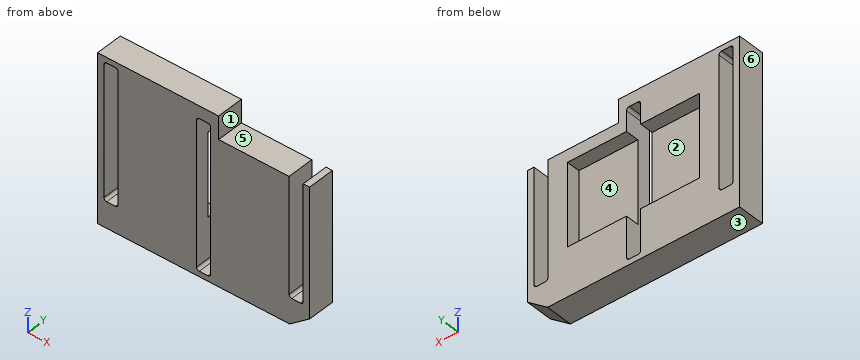
```python
from build123d import *

# Parameters (mm, degrees)
BOSS_EXTRUDE1_DEPTH = 10
FILLET1_R           = 1
SKETCH2_W           = 21.86553483
SKETCH2_H           = 30.5
CUT_EXTRUDE1_DEPTH  = 5
MIRROR1_DEPTH       = 10
MIRROR1_2_OUTLINE_W = 21.86553483
MIRROR1_2_OUTLINE_H = 30.5
MIRROR1_2_DEPTH     = 5
SKETCH6_W           = 43.680332617
SKETCH6_H           = 16.249834628
CUT_EXTRUDE2_DEPTH  = 10


# Read off the part's stored shape, not the designer's step: Mirror1
with BuildPart() as part:
    # Sketch1 → Boss-Extrude1 (new body)
    with BuildSketch(Plane(origin=(0, 0, 0), x_dir=(1, 0, 0), z_dir=(0, 1, 0))):
        Polygon((-5, 57.097150921), (34.3, 57.097150921), (34.3, 55.097150921), (31.675, 55.097150921), (31.675, 52.597150921), (31.675, 2.599340873), (31.675, 0.099340873), (34.3, 0.099340873), (34.3, -4.5), (-5, -4.5), align=None)
        Polygon((-2.625, 45), (-2.625, 0), (-2.625, -2.5), (0, -2.5), (2.625, -2.5), (2.625, 0), (2.625, 45), (2.625, 47.5), (0, 47.5), (-2.625, 47.5), align=None, mode=Mode.SUBTRACT)
    extrude(amount=BOSS_EXTRUDE1_DEPTH)

    # Fillet1
    fillet1_edges = [part.edges().sort_by_distance(p)[0] for p in [
        (31.675, 5, -55.097150921),
        (31.675, 5, -0.099340873),
        (-2.625, 5, -47.5),
        (-2.625, 5, 2.5),
        (2.625, 5, 2.5),
        (2.625, 5, -47.5),
    ]]
    fillet(fillet1_edges, radius=FILLET1_R)

    # Sketch2 → Cut-Extrude1 (cut)
    with BuildSketch(Plane(origin=(0, 10, 0), x_dir=(1, 0, 0), z_dir=(0, 1, 0))):
        with Locations((20.742232585, 23.8519351)):
            Rectangle(SKETCH2_W, SKETCH2_H)
    extrude(amount=-CUT_EXTRUDE1_DEPTH, mode=Mode.SUBTRACT)

    # Mirror1 outline → Mirror1 (add)
    with BuildSketch(Plane(origin=(0, 0, 0), x_dir=(1, 0, 0), z_dir=(0, 1, 0))):
        with BuildLine():
            ThreePointArc((35.925, 55.097150921), (36.632106781, 54.804257702), (36.925, 54.097150921))
            Line((36.925, 54.097150921), (36.925, 39.1019351))
            Line((36.925, 39.1019351), (58.79053483, 39.1019351))
            Line((58.79053483, 39.1019351), (58.79053483, 8.6019351))
            Line((58.79053483, 8.6019351), (36.925, 8.6019351))
            Line((36.925, 8.6019351), (36.925, 1.099340873))
            ThreePointArc((36.925, 1.099340873), (36.632106781, 0.392234092), (35.925, 0.099340873))
            Line((35.925, 0.099340873), (34.3, 0.099340873))
            Line((34.3, 0.099340873), (34.3, -4.5))
            Line((34.3, -4.5), (73.6, -4.5))
            Line((73.6, -4.5), (73.6, 57.097150921))
            Line((73.6, 57.097150921), (34.3, 57.097150921))
            Line((34.3, 57.097150921), (34.3, 55.097150921))
            Line((34.3, 55.097150921), (35.925, 55.097150921))
        make_face()
        with BuildLine():
            Line((70.225, -2.5), (66.975, -2.5))
            ThreePointArc((66.975, -2.5), (66.267893219, -2.207106781), (65.975, -1.5))
            Line((65.975, -1.5), (65.975, 46.5))
            ThreePointArc((65.975, 46.5), (66.267893219, 47.207106781), (66.975, 47.5))
            Line((66.975, 47.5), (70.225, 47.5))
            ThreePointArc((70.225, 47.5), (70.932106781, 47.207106781), (71.225, 46.5))
            Line((71.225, 46.5), (71.225, -1.5))
            ThreePointArc((71.225, -1.5), (70.932106781, -2.207106781), (70.225, -2.5))
        make_face(mode=Mode.SUBTRACT)
    extrude(amount=MIRROR1_DEPTH)

    # Mirror1 2 outline → Mirror1 2 (add)
    with BuildSketch(Plane(origin=(0, 0, 0), x_dir=(1, 0, 0), z_dir=(0, 1, 0))):
        with Locations((47.857767415, 23.8519351)):
            Rectangle(MIRROR1_2_OUTLINE_W, MIRROR1_2_OUTLINE_H)
    extrude(amount=MIRROR1_2_DEPTH)

    # Sketch6 → Cut-Extrude2 (cut)
    with BuildSketch(Plane(origin=(0, 10, 0), x_dir=(1, 0, 0), z_dir=(0, 1, 0))):
        with Locations((61.699631479, -4.127511542)):
            Rectangle(SKETCH6_W, SKETCH6_H)
        Polygon((66.193799085, 57.097150921), (73.6, 51.534362723), (73.6, 57.097150921), align=None)
    extrude(amount=-CUT_EXTRUDE2_DEPTH, mode=Mode.SUBTRACT)


solid = part.part
```
For this review, take the finished solid that the model builds, in its own axes (mm). Face numbers are marked on the shaded views. A direction names the side the tool comes from. Coordinates: 2 decimals unless noted, no trailing zeros. Loops run counter-clockwise (first coordinate to the right, second up) from the corner with the lowest first, then second, coordinate; pieces in that order, holes last. Notation, with made-up numbers: (-15.75, -34) - (19.25, -34) arc R34 cw to (19.25, 0) - close; hole circle Ø8 at (69.25, 70.25). An arc over 180 degrees is marked (long way). Use one line per item in the form item = value. Start each with the question number.
1) Take a section at C-C (y = 1). State how many separate pieces and enclosed holes the cut face has, plus the area to 3 significant figures.
2) For pin 1 (24 mm diameter, centred on x = 22.5, z = -25, fed in from +Y), flat-tipped, find the tip position at first contact; note if it passes through.
3) For the marked faces 4, 5 and 6, list the 3-axis set-ups (+Z, -Z, +X, -X, +Y, -Y) from which the entire face can be reached by the end or side of a thin tool; tool diameter is ignored.
4) Take a section at A-A (z = -7.5). State the section outline as (x, y) points (3 decimals), plus the area to 4 significant figures.
5) To check wall thickness, follow probe 1 along X at (y, z) = (3, -8) (3 decimals); probe 2 along X at (y, z) = (9.5, -20) (3 decimals); probe 3 along X at (y, z) = (7, -3.5) (3 decimals). State the ranges of each line that lie inside material, in increasing order. Write a range as from..to.
6) Draft analysis for pull direction Z (two halves, no side actions). For the marked faces 1, 2 and 3, state which applies: released by +Z, released by -Z, zero draft, split by the parting line, or undercut.
7) Take a section at D-D (z = -18). State the section outline as (x, y) points (3 decimals).
8) Take a section at B-B (x = 50). State the section outline as (y, z) points.
From the geometry:
q1.separate_pieces = 1
q1.enclosed_holes = 2
q1.area = 3,760 mm2
q2.pin_1 = 5
q3.face_4 = +Y
q3.face_5 = +Z, +X, +Y, -Y
q3.face_6 = +Z, -Z, -X, +Y, -Y
q4.outline = (-5, 0) - (-2.625, 0) - (-2.625, 10) - (-5, 10) - close; (2.625, 0) - (31.675, 0) - (31.675, 10) - (2.625, 10) - close; (36.925, 0) - (65.975, 0) - (65.975, 10) - (36.925, 10) - close; (71.225, 0) - (73.6, 0) - (73.6, 10) - (71.225, 10) - close
q4.area = 628.5 mm2
q5.probe_1 = -5..-2.625, 2.625..31.675, 36.925..65.975, 71.225..73.6
q5.probe_2 = -5..-2.625, 2.625..9.809, 58.791..65.975, 71.225..73.6
q5.probe_3 = -5..-2.625, 2.625..31.675, 36.925..39.859
q6.face_1 = zero draft
q6.face_2 = undercut
q6.face_3 = released by -Z
q7.outline = (-5, 0) - (-2.625, 0) - (-2.625, 10) - (-5, 10) - close; (2.625, 0) - (31.675, 0) - (31.675, 5) - (9.809, 5) - (9.809, 10) - (2.625, 10) - close; (36.925, 0) - (65.975, 0) - (65.975, 10) - (58.791, 10) - (58.791, 5) - (36.925, 5) - close; (71.225, 0) - (73.6, 0) - (73.6, 10) - (71.225, 10) - close
q8.outline = (0, -57.1) - (10, -57.1) - (10, -39.1) - (5, -39.1) - (5, -8.6) - (10, -8.6) - (10, -4) - (0, -4) - close
